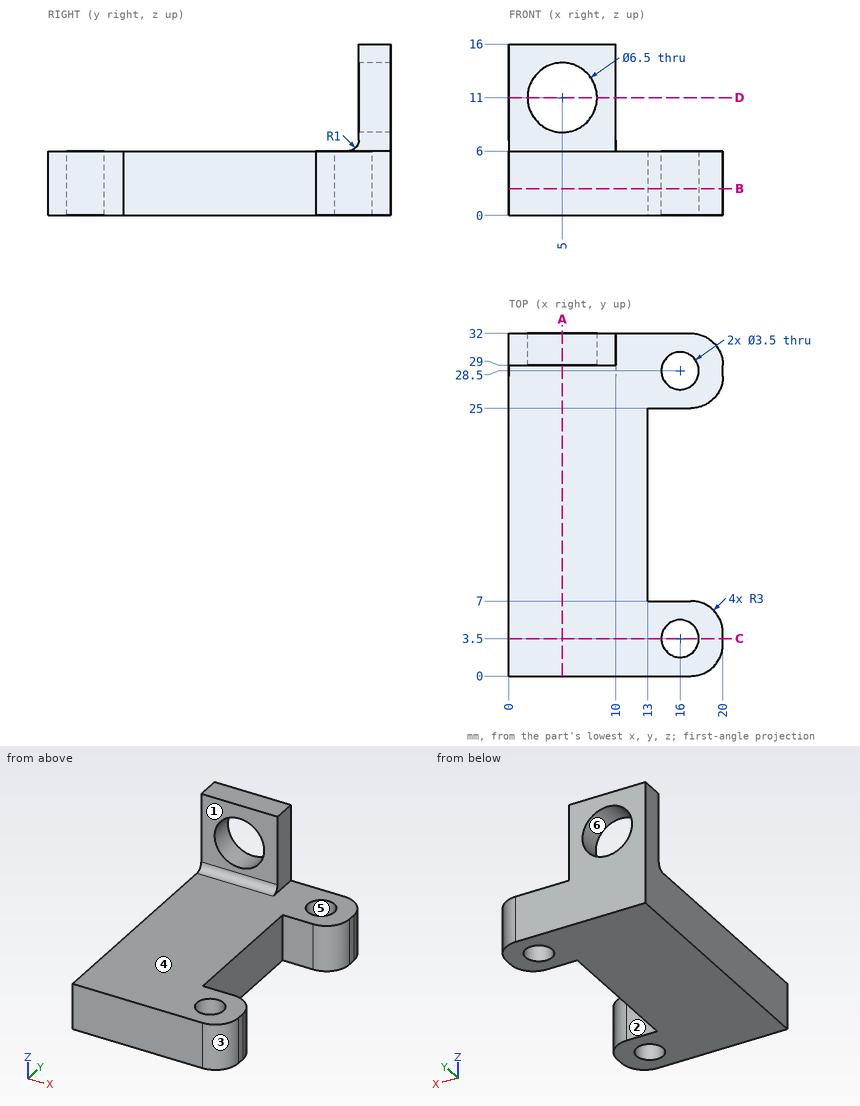
The figure shows three views and two pictorial views of one solid part (mm, origin at its lowest corner). Answer the questions. A direction names the side the tool comes from. Coordinates: 2 decimals unless noted, no trailing zeros. Loops run counter-clockwise (first coordinate to the right, second up) from the corner with the lowest first, then second, coordinate; pieces in that order, holes last. Notation, with made-up numbers: M 12,63 L 58,63 A15 cw 58,70 Z; hole C 9.25,-7 d6. An arc over 180 degrees is marked long. Use CSV: the item, a comma, the result in double quotes. Start each with the question number.
(1) Find section C-C, the plane y = 3.5. Give the vertices of the cut face in (x, z), then the cut area to 3 significant figures.
(2) Find section A-A, the plane x = 5. Give the vertices of the cut face in (y, z), then the cut area to 3 significant figures.
(3) Find section B-B, the plane z = 2.5. Give the vertices of the cut face in (x, y).
(4) For the marked faces 1, 2 and 3, determine the directions among +Z, -Z, +X, -X, +Y, -Y from which every point of the face is accessible in a straight line to the end or side of a thin tool.
(5) Consider line 1 (Y direction, x = 16, z = 3.6); line 2 (Y direction, x = 13.75, z = 3); line 3 (Z direction, x = 5, y = 31.15). Determine where each line is inside the solid, lowest interval first.
(6) For a pull along Z with two mould halves and no side action, classify the marked faces 4, 5 and 6 as +Z half, -Z half, draft (parallel to the pull), parting line (faces both ways), or undercut.
(7) Find section D-D, the plane z = 11. Give the vertices of the cut face in (x, y), then the cut area to 3 significant figures.
(8) Given pin 1 Ø1.8 at (y, z) = (20, 4) entering from +X; pin 2 Ø12 at (x, y) = (17.5, 13) entering from +Z; pin 3 Ø5 at (x, z) = (2.5, 9) entering from -Y, each flat-ended and moving along its own axis, determine where each tip first touches the part or whether it passes through.
Recorded:
1,outline,"M 0,0 L 14.25,0 L 14.25,6 L 0,6 Z; M 17.75,0 L 20,0 L 20,6 L 17.75,6 Z"
1,area,"99.0 mm^2"
2,outline,"M 0,0 L 32,0 L 32,7.75 L 29,7.75 L 29,7 A1 cw 28,6 L 0,6 Z; M 29,14.25 L 32,14.25 L 32,16 L 29,16 Z"
2,area,"203 mm^2"
3,outline,"M 0,0 L 17,0 A3 ccw 20,3 L 20,4 A3 ccw 17,7 L 13,7 L 13,25 L 17,25 A3 ccw 20,28 L 20,29 A3 ccw 17,32 L 0,32 Z; hole C 16,3.5 d3.5; hole C 16,28.5 d3.5"
4,face 1,"+Z, +X, -X, -Y"
4,face 2,"+Z, -Z, +X"
4,face 3,"+Z, -Z, +X, -Y"
5,line 1,"y = 0 to 1.75, 5.25 to 7, 25 to 26.75, 30.25 to 32"
5,line 2,"y = 0 to 7, 25 to 32"
5,line 3,"z = 0 to 7.75, 14.25 to 16"
6,face 4,"+Z half"
6,face 5,"draft"
6,face 6,"undercut"
7,outline,"M 0,29 L 1.75,29 L 1.75,32 L 0,32 Z; M 8.25,29 L 10,29 L 10,32 L 8.25,32 Z"
7,area,"10.5 mm^2"
8,pin 1,"stops at x = 13"
8,pin 2,"stops at z = 6"
8,pin 3,"stops at y = 28.87"
